Autodesk Inventor part; units mm, degrees
ref_plane "YZ Plane" through (0, 0, 0) normal (1, 0, 0) x (0, 1, 0)
ref_plane "XZ Plane" through (0, 0, 0) normal (0, 1, 0) x (-1, 0, 0)
ref_plane "XY Plane" through (0, 0, 0) normal (0, 0, 1) x (1, 0, 0)
sketch "Skizze1" plane through (0, 0, 0) normal (0, 1, 0) x (-1, 0, 0)
  line L0 (42.3, 0) -> (0, 0)
  line L1 (0, 0) -> (0, -110)
  line L2 (0, -110) -> (42.3, -110)
  line L3 (42.3, -110) -> (42.3, 0)
  dimension "d0" = 110
  dimension "d1" = 42.3
extrude "Extrusion1" add sketch "Skizze1" along normal blind 3
sketch "Skizze2" plane through (0, 3, 0) normal (0, 1, 0) x (1, 0, 0)
  line L0 (-42.3, 110) -> (-42.3, 0)
  line L1 (-42.3, 55) -> (0, 55)
  line L2 (0, 0) -> (0, 110)
  line L3 (-42.3, 0) -> (0, 0)
  line L4 (-21.15, 0) -> (-21.15, 110)
  line L5 (0, 110) -> (-42.3, 110)
  circle A0 centre (-21.15, 55) radius 11
  line L6 (-22.1428, 55) -> (16.9767, 55)
  dimension "d4" = 22
extrude "Extrusion2" cut sketch "Skizze2" against normal blind 4 contours A0 L4 L1 | L1 L4 A0 | A0 L1 L4 | L4 L1 A0
sketch "Skizze3" plane through (0, 3, 0) normal (0, 1, 0) x (1, 0, 0)
  line L0 (-42.3, 110) -> (-42.3, 0)
  line L1 (0, 0) -> (0, 110)
  line L2 (-42.3, 0) -> (0, 0)
  line L3 (-21.15, 0) -> (-21.15, 110)
  line L4 (0, 110) -> (-42.3, 110)
  circle A0 centre (-21.15, 55) radius 21.9203 construction
  line L5 (-21.15, 55) -> (-36.65, 55) construction
  line L6 (-36.65, 39.5) -> (-36.65, 70.5) construction
  circle A1 centre (-36.65, 39.5) radius 1.75
  circle A2 centre (-36.65, 70.5) radius 1.75
  circle A3 centre (-5.65, 39.5) radius 1.75
  circle A4 centre (-5.65, 70.5) radius 1.75
  dimension "d7" = 15.5
  dimension "d8" = 31
  dimension "d9" = 3.5
  dimension "d10" = 3.5
extrude "Extrusion3" cut sketch "Skizze3" against normal blind 4 contours A1 | A2 | A3 | A4
sketch "Skizze4" plane through (-45.3, -3, -110) normal (-1, 0, 0) x (0, -1, 0)
  line L0 (0, 110) -> (0, 0)
  line L1 (0, 0) -> (14, 0)
  line L2 (14, 0) -> (14, 110)
  line L3 (14, 110) -> (0, 110)
edge flange "Lasche1" height 20 angle 90 thickness 3 bend radius 3 thickness toward (-1, 0, 0) relief tear relief width 3 relief depth 1.5 edges at (-42.3, 0, -55) wall of the first edge with corners at (-45.3, -3, 0) (-45.3, -3, -110) (-45.3, -17, -110) (-45.3, -17, 0)
bend "Biegung1"
corner "Ecke1"
sketch "Skizze5" plane through (3, -3, 0) normal (1, 0, 0) x (0, 1, 0)
  line L0 (0, -110) -> (0, 0)
  line L1 (0, 0) -> (-14, 0)
  line L2 (-14, 0) -> (-14, -110)
  line L3 (-14, -110) -> (0, -110)
edge flange "Lasche2" height 20 angle 90 thickness 3 bend radius 3 thickness toward (1, 0, 0) relief tear relief width 3 relief depth 1.5 edges at (0, 0, -55) wall of the first edge with corners at (3, -3, -110) (3, -3, 0) (3, -17, 0) (3, -17, -110)
bend "Biegung2"
corner "Ecke2"
sketch "Skizze6" plane through (6, -17, 0) normal (1, 0, 0) x (0, 0, -1)
  line L0 (0, 0) -> (0, 14)
  line L1 (0, 7) -> (110, 7)
  line L2 (110, 0) -> (110, 14)
  line L3 (110, 0) -> (0, 0)
  line L4 (55, 0) -> (55, 14)
  line L5 (0, 14) -> (110, 14)
  circle A0 centre (67.5, 7) radius 2.25
  circle A1 centre (42.5, 7) radius 2.25
  circle A2 centre (95, 7) radius 2.25
  circle A3 centre (15, 7) radius 2.25
  point P0 (0, 17)
  point P1 (17.25, 7)
  point P2 (12.75, 7)
  dimension "d35" = 4.5
  dimension "d36" = 4.5
  dimension "d37" = 25
  dimension "d41" = 4.5
  dimension "d42" = 4.5
  dimension "d43" = 80
fillet "Rundung2" radius 2 4 edges at (-46.8, -17, -110) (4.5, -17, -110) (-46.8, -17, 0) (4.5, -17, 0)
extrude "Extrusion5" cut sketch "Skizze6" against normal blind 100 contours A3 L1 | L1 A3 | A1 L1 | L1 A1 | A0 L1 | L1 A0 | A2 L1 | L1 A2
equation "\"d14\" = Stärke"
equation "\"d15\" = BreiteBiegungsfreistellung"
equation "\"d16\" = TiefeBiegungsfreistellung"
equation "\"d17\" = MinimalRest"
equation "\"d18\" = Übergangsradius"
equation "\"d21\" = Biegeradius"
equation "\"d22\" = GrößeEckenfreistellung"
equation "\"d23\" = Abstandsgröße"
equation "\"d24\" = JacobiRadiusGröße"
equation "\"d25\" = BreiteBiegungsfreistellung"
equation "\"d26\" = TiefeBiegungsfreistellung"
equation "\"d27\" = MinimalRest"
equation "\"d28\" = Übergangsradius"
equation "\"d31\" = Biegeradius"
equation "\"d32\" = GrößeEckenfreistellung"
equation "\"d33\" = Abstandsgröße"
equation "\"d34\" = JacobiRadiusGröße"
equation "\"Biegeradius\" = Stärke"
equation "\"BreiteBiegungsfreistellung\" = Stärke"
equation "\"TiefeBiegungsfreistellung\" = 0.5 * Stärke"
equation "\"GrößeEckenfreistellung\" = 4 * Stärke"
equation "\"MinimalRest\" = 2 * Stärke"
equation "\"Übergangsradius\" = Biegeradius"
equation "\"JacobiRadiusGröße\" = Biegeradius"
equation "\"Abstandsgröße\" = Stärke"
properties part number "Motorhalter_02" material "Aluminium 6061"
CAD build for the part. Positions are in the model's coordinates, mm. A direction names the side the tool comes from. Round coordinates to 2 decimals unless told otherwise and drop trailing zeros. Write each loop counter-clockwise with the first axis right and the second up, starting at its lowest first coordinate (ties: lowest second). Pieces come first, ordered by that corner, then holes. Notation, with made-up numbers: (86.25, -15) - (109.25, -15) arc R14 ccw to (109.25, 4) - close; hole circle Ø9 at (-32, 58.5). An arc over 180 degrees is marked (long way). Write item = value, one per line. Start each with the question number.
Q1. Band-saw the part on B-B (x = -5.65). Give the cut face in (y, z), then the cut area to 3 significant figures.
Q2. Band-saw the part on D-D (z = -42.5). Give the cut face in (x, y), then the cut area to 3 significant figures.
Q3. Mould opens along X. For faces 3 (the flat face through (-48.3, -10, -56)), 4 (the flat face through (-45.3, -10, -56)), 5 (the cylindrical face through (4.521, -9.901, -40.252)) say: pulls with the +X half, pulls with the -X half, needs draft (parallel to the pull), parting line crosses it, or undercut.
Q4. Drop flat-ended pins along their axis: pin 1 (4 mm diameter, centred on x = -36.65, z = -70.5, fed in from +Y); pin 2 (21 mm diameter, centred on x = -26.5, z = -70.5, fed in from -Y); pin 3 (3 mm diameter, centred on x = -36.65, z = -39.5, fed in from +Y). Give the stop position or say it passes through.
Q5. Band-saw the part on C-C (y = -5). Give the cut face in (x, z).
Q6. Band-saw the part on A-A (z = -55). Give the cut face in (x, y).
Q7. Which spindle directions (+Z, -Z, +X, -X, +Y, -Y) get a long thin tool onto all of the face, cutting with end or side? Do faces 1 (the cylindrical face through (2.14, -0.9, -54.23)), 2 (the cylindrical face through (-46.82, -16.43, -0.6)). Say none if no direction does.
Q8. Probe L1, parallel to Z at x = -5.65, y = 1; L2, parallel to X at y = -10.25, z = -104.5; L3, parallel to Z at x = 4, y = -8. List the from-to ranges inside material, lowest first. Write a range as from..to.
Answers below:
q1.outline = (0, -110) - (3, -110) - (3, -72.25) - (0, -72.25) - close; (0, -68.75) - (3, -68.75) - (3, -41.25) - (0, -41.25) - close; (0, -37.75) - (3, -37.75) - (3, 0) - (0, 0) - close
q1.area = 309 mm2
q2.outline = (-48.3, -17) - (-45.3, -17) - (-45.3, -12.25) - (-48.3, -12.25) - close; (-48.3, -7.75) - (-45.3, -7.75) - (-45.3, -3) arc R3 cw to (-42.3, 0) - (0, 0) arc R3 cw to (3, -3) - (3, -7.75) - (6, -7.75) - (6, -3) arc R6 ccw to (0, 3) - (-42.3, 3) arc R6 ccw to (-48.3, -3) - close; (3, -17) - (6, -17) - (6, -12.25) - (3, -12.25) - close
q2.area = 226 mm2
q3.face_3 = pulls with the -X half
q3.face_4 = undercut
q3.face_5 = needs draft
q4.pin_1 = 3
q4.pin_2 = 0
q4.pin_3 = through
q5.outline = (-48.3, -110) - (-45.3, -110) - (-45.3, 0) - (-48.3, 0) - close; (3, -110) - (6, -110) - (6, 0) - (3, 0) - close
q6.outline = (-48.3, -17) - (-45.3, -17) - (-45.3, -3) arc R3 cw to (-42.3, 0) - (-32.15, 0) - (-32.15, 3) - (-42.3, 3) arc R6 ccw to (-48.3, -3) - close; (-10.15, 0) - (0, 0) arc R3 cw to (3, -3) - (3, -17) - (6, -17) - (6, -3) arc R6 ccw to (0, 3) - (-10.15, 3) - close
q7.face_1 = +Z, -Z, -Y
q7.face_2 = +Z, +X, -X, -Y
q8.L1 = -110..-72.25, -68.75..-41.25, -37.75..0
q8.L2 = -48.3..-45.3, 3..6
q8.L3 = -110..-96.03, -93.97..-68.53, -66.47..-43.53, -41.47..-16.03, -13.97..0
